```python
from build123d import *

# Parameters (mm, degrees)
F0_R     = 11
F1_DEPTH = 5
F2_R     = 4.5
F3_DEPTH = 12
F5_DEPTH = 4.5
F6_R     = 2
F8_D     = 5
F8_DEPTH = 14.4
F8_TIP   = 1.5021515476


with BuildPart() as f1:
    # F0 (on Top) → F1 (new body)
    with BuildSketch(Plane.XY):
        Circle(F0_R)
    extrude(amount=F1_DEPTH)

    # F2 (on face) → F3 (join)
    with BuildSketch(Plane.XY.offset(5)):
        Circle(F2_R)
    extrude(amount=F3_DEPTH)

    # F4 (on Front) → F5 (join, symmetric)
    with BuildSketch(Plane.XZ):
        with BuildLine():
            Line((-6.9616497494, 13), (0, 13))
            Line((0, 13), (6.9616497494, 13))
            ThreePointArc((6.9616497494, 13), (9.3963810746, 11.8065304048), (9.9443754998, 9.1509723824))
            Line((9.9443754998, 9.1509723824), (14, 9.1509723824))
            ThreePointArc((14, 9.1509723824), (12.2329306372, 14.6466278196), (6.9616497494, 17))
            Line((6.9616497494, 17), (0, 17))
            Line((0, 17), (-6.9616497494, 17))
            ThreePointArc((-6.9616497494, 17), (-12.2329306372, 14.6466278196), (-14, 9.1509723824))
            Line((-14, 9.1509723824), (-9.9443754998, 9.1509723824))
            ThreePointArc((-9.9443754998, 9.1509723824), (-9.3963810746, 11.8065304048), (-6.9616497494, 13))
        make_face()
    extrude(amount=F5_DEPTH, both=True)

    # F6
    f6_edges = [f1.edges().sort_by_distance(p)[0] for p in [
        (-11, 0, 5),
        (0, -4.5, 17),
        (0, 4.5, 17),
        (-9.944375, 0, 9.150972),
        (9.944375, 0, 9.150972),
    ]]
    fillet(f6_edges, radius=F6_R)

    # F8
    with Locations(Plane(origin=(0, 0, 0), x_dir=(1, 0, 0), z_dir=(0, 0, -1))):
        with Locations((0, 0)):
            Hole(F8_D / 2, depth=F8_DEPTH)
            with Locations((0, 0, -(F8_DEPTH + F8_TIP / 2))):  # 118° drill point
                Cone(0, F8_D / 2, F8_TIP, mode=Mode.SUBTRACT)


solid = f1.part
```
The model under review builds one solid part; all positions refer to its coordinate system, in mm. A direction names the side the tool comes from. Round coordinates to 2 decimals unless told otherwise and drop trailing zeros. Order: outer loops, then holes, each group sorted by start corner. A loop starts at its lowest first (then second) coordinate and runs counter-clockwise, first axis right, second up. Notation, with made-up numbers: (40, 2.25) -> (65, 2.25) arc R30 ccw to (65, 29.25) -> close; hole circle Ø6 at (79, 68.25). An arc over 180 degrees is marked (long way). One line per item, written item: value. Start each with the question number.
Q1. Clearance check with flat-ended pins moving along their axes: pin 1 Ø6.5 at (x, z) = (3.5, 12) entering from +Y; pin 2 Ø8 at (x, y) = (-6.5, 5) entering from +Z; pin 3 Ø2.5 at (x, y) = (13, 1) entering from -Z; pin 4 Ø1.8 at (x, z) = (-1.5, 12.5) entering from -Y. State where each tip first meets the part, or that it passes through.
Q2. Take a section at A-A (z = 12). Count the separate pieces of the cut face and the enclosed holes in it, and give its area (3 significant figures).
Q3. Take a section at B-B (z = 3.75). Write out the cut boundary in (x, y), and give its area (3 significant figures).
Q4. Mouldability with a two-part tool opening along Z and no side actions: class faces 6 (the face through (-3, 0, 0)), 7 (the face through (-2.38, -10.74, 1.48)), 8 (the face through (-0.59, 4.46, 8.94)) as released by +Z, released by -Z, zero draft, split by the parting line, or undercut.
Q5. Machinability: for faces 1 (the face through (-5, 0, 13)), 2 (the face through (8.835, -0.063, 12.365)), 3 (the face through (-13, 0, 9.151)), 4 (the face through (0.54, 2.44, 7.3)), 5 (the face through (13, 0, 9.151)), which of the approach directions +Z, -Z, +X, -X, +Y, -Y give a long, thin tool a straight path to every point of the face, cutting with its end or side? Answer none if there is none.
Q6. Wall thickness on line 1 (Y direction, x = 0, z = 6.25); line 2 (X direction, y = 1.25, z = 10.5); line 3 (Z direction, x = -4.75, y = 2.5): over which ranges is each line inside the solid? List them lowest first.
Reported:
1. pin 1: stops at y = 4.5
1. pin 2: stops at z = 17
1. pin 3: stops at z = 9.15
1. pin 4: stops at y = -4.5
2. separate pieces: 3
2. enclosed holes: 1
2. area: 121 mm2
3. outline: circle Ø21.71 at (0, 0); hole circle Ø5 at (0, 0)
3. area: 350 mm2
4. face 6: released by -Z
4. face 7: zero draft
4. face 8: undercut
5. face 1: none
5. face 2: +Y, -Y
5. face 3: -Z, -X, +Y, -Y
5. face 4: -Z
5. face 5: -Z, +X, +Y, -Y
6. line 1: y = -4.5 to -2.5, 2.5 to 4.5
6. line 2: x = -14.02 to -10, -4.32 to -2.17, 2.17 to 4.32, 10 to 14.02
6. line 3: z = 0 to 5, 13 to 17
